Answer from the drawing. Dimensions are ordinates in mm from the lowest x, y and z of the part. A direction names the side the tool comes from. Coordinates: 2 decimals unless noted, no trailing zeros. Order: outer loops, then holes, each group sorted by start corner. A loop starts at its lowest first (then second) coordinate and runs counter-clockwise, first axis right, second up. Notation, with made-up numbers: (-10.75, -4.5) -> (46.25, -4.5) arc R17 cw to (46.25, 21.5) -> close; hole circle Ø3 at (-3.75, -21.5). An arc over 180 degrees is marked (long way). Use CSV: the item, a comma, the result in double quotes.
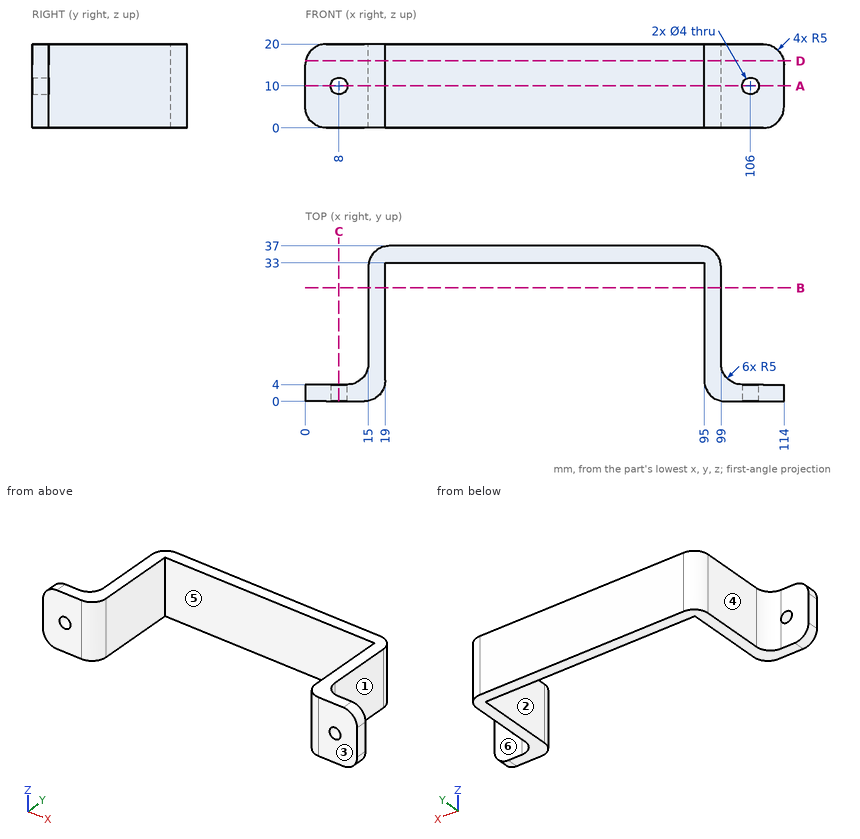
Item 1: Find section D-D, the plane z = 16. Give the vertices of the cut face in (x, y), then the cut area to 3 significant figures.
Return value:
outline,"(0.1, 0) -> (14, 0) arc R5 ccw to (19, 5) -> (19, 33) -> (95, 33) -> (95, 5) arc R5 ccw to (100, 0) -> (113.9, 0) -> (113.9, 4) -> (104, 4) arc R5 cw to (99, 9) -> (99, 32) arc R5 ccw to (94, 37) -> (20, 37) arc R5 ccw to (15, 32) -> (15, 9) arc R5 cw to (10, 4) -> (0.1, 4) -> close"
area,"708 mm^2"
Item 2: The mould has two halves that part along X. Classify the marked faces 1, 2 and 3: +X half, -X half, draft (parallel to the pull), parting line (faces both ways), or undercut.
Return value:
face 1,"+X half"
face 2,"undercut"
face 3,"draft"
Item 3: Find section B-B, the plane y = 27. Give the vertices of the cut face in (x, z).
Return value:
outline,"(15, 0) -> (19, 0) -> (19, 20) -> (15, 20) -> close; (95, 0) -> (99, 0) -> (99, 20) -> (95, 20) -> close"
Item 4: Straight lines are drawn through the part: line 1 along X through (y, z) = (24.5, 7.25); line 2 along Z through (x, y) = (8, 1.9); line 3 along Y through (x, z) = (22.5, 10.5). For each, find the intervals that lie inside material, in ascending order.
Return value:
line 1,"x = 15 to 19, 95 to 99"
line 2,"z = 0 to 8, 12 to 20"
line 3,"y = 33 to 37"
Item 5: Find section A-A, the plane z = 10. Give the number of separate pieces and of enclosed holes in the cut face, then the cut area to 3 significant figures.
Return value:
separate pieces,"3"
enclosed holes,"0"
area,"677 mm^2"
Item 6: Find section C-C, the plane x = 8. Give the vertices of the cut face in (y, z), then the cut area to 3 significant figures.
Return value:
outline,"(0, 0) -> (4, 0) -> (4, 8) -> (0, 8) -> close; (0, 12) -> (4, 12) -> (4, 20) -> (0, 20) -> close"
area,"64.0 mm^2"
Item 7: A tool of negligible diameter and unlimited length cuts with its end or side. For the marked faces 4, 5 and 6, from which of +Z, -Z, +X, -X, +Y, -Y can it reach the whole face along a straight path? Write none if from no direction.
Return value:
face 4,"+Z, -Z, -X, +Y"
face 5,"+Z, -Z, -Y"
face 6,"+Z, -Z, +X, +Y"
Item 8: Each of these flat-tipped pins is pushed along its axis until it touches: P1, Ø8, axis at x = 110.5, z = 11, coming from the +Y side; P2, Ø10, axis at y = 26, z = 10, coming from the +X side; P3, Ø12, axis at y = 20.5, z = 4.5, coming from the -X side. Where does it stop, or does it pass through?
Return value:
P1,"stops at y = 4"
P2,"stops at x = 99"
P3,"stops at x = 15"
